```python
from build123d import *

# Parameters (mm, degrees)
F0_W     = 62
F0_H     = 62
F1_DEPTH = 21
F2_W     = 62
F2_H     = 17
F3_DEPTH = 60
F4_W     = 60
F4_H     = 17
F5_DEPTH = 62


with BuildPart() as f1:
    # F0 (on Top) → F1 (new body)
    with BuildSketch(Plane.XY):
        with Locations((62, 0)):
            Rectangle(F0_W, F0_H)
        Rectangle(F0_W, F0_H)
        with Locations((0, -62)):
            Rectangle(F0_W, F0_H)
    extrude(amount=F1_DEPTH)

    # F2 (on face) → F3 (cut)
    with BuildSketch(Plane.YZ.offset(31)):
        with Locations((-62, 10.5)):
            Rectangle(F2_W, F2_H)
    extrude(amount=-F3_DEPTH, mode=Mode.SUBTRACT)

    # F4 (on face) → F5 (cut)
    with BuildSketch(Plane.YZ.offset(93)):
        with Locations((-1, 10.5)):
            Rectangle(F4_W, F4_H)
    extrude(amount=-F5_DEPTH, mode=Mode.SUBTRACT)


solid = f1.part
```
The model under review builds one solid part; all positions refer to its coordinate system, in mm. A direction names the side the tool comes from. Round coordinates to 2 decimals unless told otherwise and drop trailing zeros. Loops run counter-clockwise (first coordinate to the right, second up) from the corner with the lowest first, then second, coordinate; pieces in that order, holes last.
Item 1: Mouldability with a two-part tool opening along Z and no side actions: class faces 3 (the face through (1, -31, 10)), 4 (the face through (16, -16, 21)), 5 (the face through (-31, -30, 10)), 6 (the face through (16, -16, 0)) as released by +Z, released by -Z, zero draft, split by the parting line, or undercut.
Determined:
face 3: undercut
face 4: released by +Z
face 5: zero draft
face 6: released by -Z
Item 2: For faces 1 (the face through (1, -62, 19)), 2 (the face through (93, 2, 20)), list the 3-axis set-ups (+Z, -Z, +X, -X, +Y, -Y) from which the entire face can be reached by the end or side of a thin tool; tool diameter is ignored.
Determined:
face 1: +X, -Y
face 2: +Z, -Z, +X, +Y, -Y
Item 3: Take a section at A-A (x = 45). Write out the cut boundary in (y, z), then the cut area to 3 significant figures.
Determined:
outline: (-31, 0) - (31, 0) - (31, 21) - (-31, 21) - (-31, 19) - (29, 19) - (29, 2) - (-31, 2) - close
area: 282 mm2
Item 4: Take a section at B-B (z = 11.5). Write out the cut boundary in (x, y).
Determined:
outline: (-31, -93) - (-29, -93) - (-29, -31) - (31, -31) - (31, 29) - (93, 29) - (93, 31) - (-31, 31) - close
Item 5: For line 1 (Z direction, x = 75, y = 4); line 2 (Y direction, x = 65.5, z = 16.5); line 3 (X direction, y = -40, z = 4.5), list the stretches that pass through material, from the lowest coordinate up.
Determined:
line 1: z = 0 to 2, 19 to 21
line 2: y = 29 to 31
line 3: x = -31 to -29
Item 6: Clearance check with flat-ended pins moving along their axes: pin 1 Ø1 at (y, z) = (-64.5, 19.5) entering from +X; pin 2 Ø2 at (x, z) = (64.5, 20) entering from -Y; pin 3 Ø5 at (x, z) = (50, 9) entering from -Y. State where each tip first meets the part, or that it passes through.
Determined:
pin 1: stops at x = 31
pin 2: stops at y = -31
pin 3: stops at y = 29
